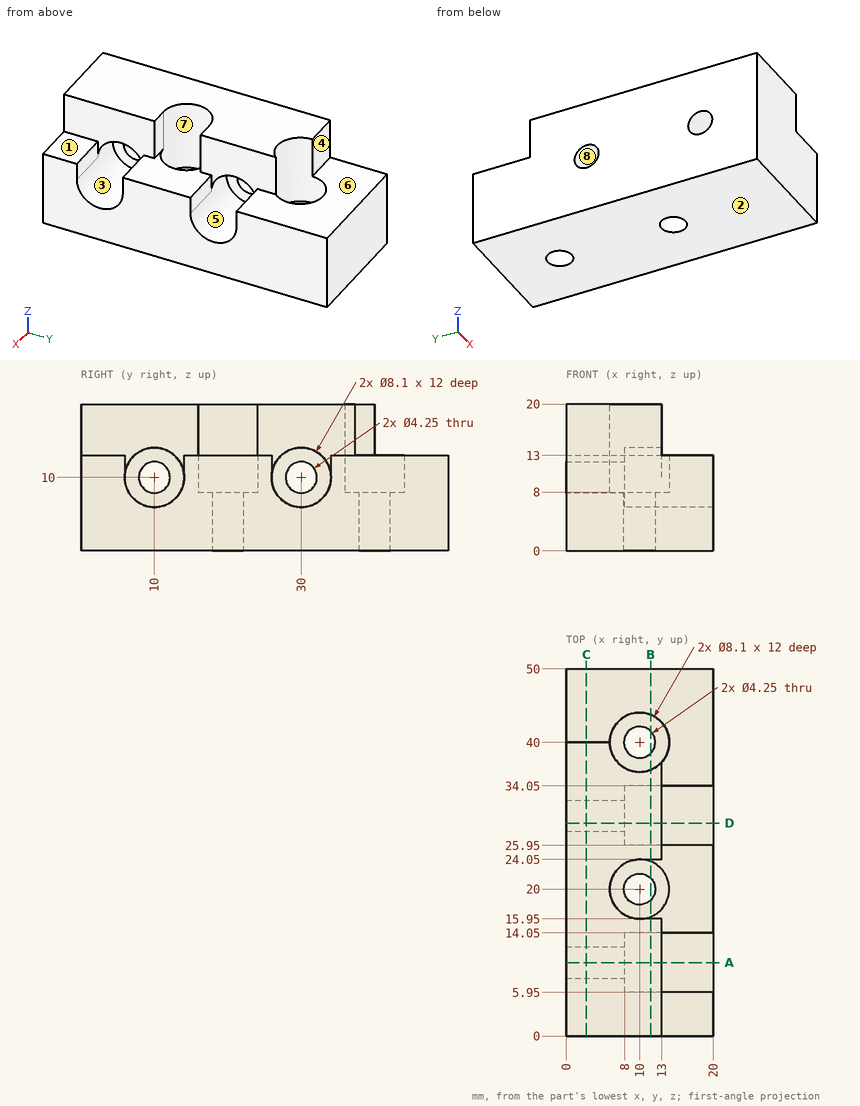
Print and shaded views of the part. All mm, measured from the part's lowest x, y and z. A direction names the side the tool comes from. Coordinates: 2 decimals unless noted, no trailing zeros. Order: outer loops, then holes, each group sorted by start corner. A loop starts at its lowest first (then second) coordinate and runs counter-clockwise, first axis right, second up. Notation, with made-up numbers: (23.25, 16) - (64.25, 16) arc R15 cw to (64.25, 45) - close; hole circle Ø3 at (58.25, 55.25). An arc over 180 degrees is marked (long way). Return JSON: item names as keys, results as strings. Group by question number.
Item 1: Pin check, flat tips, straight feed: pin 1 (5 mm diameter, centred on x = 17.5, y = 37.5, fed in from +Z); pin 2 (5 mm diameter, centred on x = 2.5, z = 17.5, fed in from +Y); pin 3 (3.5 mm diameter, centred on y = 10, z = 10, fed in from -X); pin 4 (3.5 mm diameter, centred on x = 11.5, z = 16, fed in from +Y). Stop position of each tip, or through.
Item 2: Cut at C-C (x = 2.75). List the corners of the cut face in (y, z) (3 decimals), plus the area to 3 significant figures.
Item 3: Cut at A-A (y = 10). List the corners of the cut face in (x, z) (3 decimals), plus the area to 3 significant figures.
Item 4: Cut at D-D (y = 29). List the corners of the cut face in (x, z) (3 decimals), plus the area to 3 significant figures.
Item 5: Pull direction Z, two halves, no side cores. Call the marked faces 1, 2 and 3: pulls with the +Z half, pulls with the -Z half, needs draft (parallel to the pull), parting line crosses it, or undercut.
Item 6: Drill centre lines: probe 1 along Y at (x, z) = (10, 1.75) (3 decimals); probe 2 along Y at (x, z) = (17.5, 10); probe 3 along Z at (x, y) = (10.5, 30). Where is each one in solid material? Low to high. Write a range as from..to.
Item 7: Cut at B-B (x = 11.5). List the corners of the cut face in (y, z), plus the area to 4 significant figures.
Item 8: Which spindle directions (+Z, -Z, +X, -X, +Y, -Y) get a long thin tool onto all of the face, cutting with end or side? Do the marked faces 4, 5, 6, 7 and 8. Say none if no direction does.
Check values:
{
 "1": {"pin 1": "stops at z = 13", "pin 2": "stops at y = 40", "pin 3": "passes through", "pin 4": "stops at y = 37.28"},
 "2": {"outline": "(0, 0) - (50, 0) - (50, 13) - (40, 13) - (40, 20) - (0, 20) - close; hole circle Ø4.25 at (10, 10); hole circle Ø4.25 at (30, 10)", "area": "902 mm2"},
 "3": {"outline": "(0, 0) - (20, 0) - (20, 5.95) - (8, 5.95) - (8, 7.875) - (0, 7.875) - close; (0, 12.125) - (8, 12.125) - (8, 14.05) - (13, 14.05) - (13, 20) - (0, 20) - close", "area": "227 mm2"},
 "4": {"outline": "(0, 0) - (20, 0) - (20, 6.075) - (8, 6.075) - (8, 8.125) - (0, 8.125) - close; (0, 11.875) - (8, 11.875) - (8, 13.925) - (13, 13.925) - (13, 20) - (0, 20) - close", "area": "233 mm2"},
 "5": {"face 1": "pulls with the +Z half", "face 2": "pulls with the -Z half", "face 3": "undercut"},
 "6": {"probe 1": "y = 0..17.875, 22.125..37.875, 42.125..50", "probe 2": "y = 0..5.95, 14.05..25.95, 34.05..50", "probe 3": "z = 0..5.95, 14.05..20"},
 "7": {"outline": "(0, 0) - (18.49, 0) - (18.49, 8) - (16.24, 8) - (16.24, 13) - (15.95, 13) - (15.95, 20) - (0, 20) - close; (21.51, 0) - (38.49, 0) - (38.49, 8) - (36.24, 8) - (36.24, 20) - (24.05, 20) - (24.05, 13) - (23.76, 13) - (23.76, 8) - (21.51, 8) - close; (41.51, 0) - (50, 0) - (50, 13) - (43.76, 13) - (43.76, 8) - (41.51, 8) - close; hole circle Ø8.1 at (10, 10); hole circle Ø8.1 at (30, 10)", "area": "620.5 mm2"},
 "8": {"face 4": "+Z, +X, -X, +Y", "face 5": "+X", "face 6": "+Z, +X, +Y", "face 7": "+Z", "face 8": "+X, -X"}
}
